```python
from build123d import *

# Parameters (mm, degrees)
DODANIE_WYCI_GNI_CIE1_DEPTH = 11.5
SZKIC2_R                    = 1
DODANIE_WYCI_GNI_CIE2_DEPTH = 10
WYTNIJ_WYCI_GNI_CIE1_DEPTH  = 10


with BuildPart() as part:
    # Szkic1 → Dodanie-wyciągnięcie1 (new body, symmetric)
    with BuildSketch(Plane.XY):
        Polygon((0, 0), (0, 14), (5.5, 14), (5.5, 6.5), (2.8, 6.5), (2.8, 0), align=None)
    extrude(amount=DODANIE_WYCI_GNI_CIE1_DEPTH, both=True)

    # Szkic2 → Dodanie-wyciągnięcie2 (add)
    with BuildSketch(Plane(origin=(0, 0, -11.5), x_dir=(-1, 0, 0), z_dir=(0, 0, -1))):
        with Locations((-2.75, 11.5)):
            Circle(SZKIC2_R)
        with Locations((-2.75, 9)):
            Circle(SZKIC2_R)
    extrude(amount=DODANIE_WYCI_GNI_CIE2_DEPTH)

    # Szkic3 → Wytnij-wyciągnięcie1 (cut)
    with BuildSketch(Plane(origin=(2.8, 0, 0), x_dir=(0, 0, -1), z_dir=(1, 0, 0))):
        with BuildLine():
            Line((-8.024695077, 1.5), (-5.975304923, 1.5))
            ThreePointArc((-5.975304923, 1.5), (-5.1, 3.1), (-5.975304923, 4.7))
            Line((-5.975304923, 4.7), (-8.024695077, 4.7))
            ThreePointArc((-8.024695077, 4.7), (-8.9, 3.1), (-8.024695077, 1.5))
        make_face()
        with BuildLine():
            Line((8.024695077, 1.5), (5.975304923, 1.5))
            ThreePointArc((5.975304923, 1.5), (5.1, 3.1), (5.975304923, 4.7))
            Line((5.975304923, 4.7), (8.024695077, 4.7))
            ThreePointArc((8.024695077, 4.7), (8.9, 3.1), (8.024695077, 1.5))
        make_face()
    extrude(amount=-WYTNIJ_WYCI_GNI_CIE1_DEPTH, mode=Mode.SUBTRACT)


solid = part.part
```
Here's how the part is built. I have some questions about the finished solid (model axes, mm). A direction names the side the tool comes from. Give positions to 0.01 mm unless a question says otherwise; leave off trailing zeros. Write each loop counter-clockwise with the first axis right and the second up, starting at its lowest first coordinate (ties: lowest second). Pieces come first, ordered by that corner, then holes. Notation, with made-up numbers: M 62.5,61 L 83.5,61 A19 cw 83.5,68 Z; hole C -22,-6 d3. An arc over 180 degrees is marked long. Put each result on its own line as item: value. Start each with the question number.
Item 1: Thinking about a two-plate mould opening in Z: for faces 1 (the flat face through (2, 9, 11.5)), 2 (the cylindrical face through (1.4, 3.1, 5.1)), 3 (the flat face through (5.5, 10, 0)), which applies, +Z half, -Z half, draft (parallel to the pull), parting line (faces both ways), or undercut?
Item 2: I need wall thicknesses on L1, parallel to Z at x = 2.65, y = 2; L2, parallel to Y at x = 2.1, z = -7; L3, parallel to X at y = 2.5, z = 2. Which ranges of each line are inside material? Lowest first, please. Write a range as from..to.
Item 3: If we section it at D-D, the plane x = 3.35: Write out the boundary of the cut face in (y, z), then the cut area to 4 significant figures.
Item 4: If we section it at A-A, the plane z = 7: Write out the boundary of the cut face in (x, y).
Item 5: If we section it at C-C, the plane y = 9: Write out the boundary of the cut face in (x, z), then the cut area to 4 significant figures.
Item 6: On a 3-axis mill with a long thin cutter (end or side, diameter ignored), from which of +Z, -Z, +X, -X, +Y, -Y can I reach the whole of each face in a straight line? I mean faces 4 (the flat face through (3, 12, -21.5)), 5 (the flat face through (2.8, 3, 0)), 6 (the cylindrical face through (1.4, 3.1, -8.9)), 7 (the cylindrical face through (3.54, 10.89, -16.43)). Say none if no direction works.
Item 7: If we section it at B-B, the plane x = 0.65: Write out the boundary of the cut face in (y, z).
Item 8: Will these pins go through, and if not, where does the flat tip stop? pin 1 (5 mm diameter, centred on y = 2.5, z = -0.5, fed in from +X); pin 2 (3 mm diameter, centred on x = 1.5, y = 3.5, fed in from -Z); pin 3 (0.6 mm diameter, centred on x = 1.5, z = -6.5, fed in from -Y); pin 4 (2 mm diameter, centred on y = 8, z = -14, fed in from +X).
Values:
1. face 1: +Z half
1. face 2: undercut
1. face 3: draft
2. L1: -11.5..-8.55, -5.45..5.45, 8.55..11.5
2. L2: 0..1.5, 4.7..14
2. L3: 0..2.8
3. outline: M 6.5,-11.5 L 8.2,-11.5 L 8.2,-21.5 L 9.8,-21.5 L 9.8,-11.5 L 10.7,-11.5 L 10.7,-21.5 L 12.3,-21.5 L 12.3,-11.5 L 14,-11.5 L 14,11.5 L 6.5,11.5 Z
3. area: 204.5 mm²
4. outline: M 0,0 L 2.8,0 L 2.8,1.5 L 0,1.5 Z; M 0,4.7 L 2.8,4.7 L 2.8,6.5 L 5.5,6.5 L 5.5,14 L 0,14 Z
5. outline: M 0,-11.5 L 1.75,-11.5 L 1.75,-21.5 L 3.75,-21.5 L 3.75,-11.5 L 5.5,-11.5 L 5.5,11.5 L 0,11.5 Z
5. area: 146.5 mm²
6. face 4: -Z, +X, -X, +Y, -Y
6. face 5: +Z, -Z, +X, -Y
6. face 6: +X, -X
6. face 7: -Z
7. outline: M 0,-11.5 L 14,-11.5 L 14,11.5 L 0,11.5 Z; hole M 1.5,-8.02 A1.9 ccw 4.7,-8.02 L 4.7,-5.98 A1.9 ccw 1.5,-5.98 Z; hole M 1.5,5.98 A1.9 ccw 4.7,5.98 L 4.7,8.02 A1.9 ccw 1.5,8.02 Z
8. pin 1: x = 2.8
8. pin 2: z = -11.5
8. pin 3: y = 0
8. pin 4: x = 3.75
